For this review, take the finished solid that the model builds, in its own axes (mm). Face numbers are marked on the shaded views. A direction names the side the tool comes from. Coordinates: 2 decimals unless noted, no trailing zeros. Order: outer loops, then holes, each group sorted by start corner. A loop starts at its lowest first (then second) coordinate and runs counter-clockwise, first axis right, second up. Notation, with made-up numbers: (87, 7) - (139, 7) arc R21 ccw to (139, 33) - close; hole circle Ø11 at (-17, 34.25). An arc over 180 degrees is marked (long way). One line per item, written item: value. Start each with the question number.
(1) To check wall thickness, follow line 1 along X through (y, z) = (-1.4, 0.55); line 2 along X through (y, z) = (0.1, -0.4); line 3 along Y through (x, z) = (4.5, 0.4). State the ranges of each line that lie inside material, in increasing order.
(2) Consider section A-A on x = 3. Write out the cut boundary in (y, z), then the cut area to 3 significant figures.
(3) Clearance check with flat-ended pins moving along their axes: pin 1 (1.5 mm diameter, centred on x = 2, z = 0.5, fed in from -Y); pin 2 (0.6 mm diameter, centred on x = 0.5, z = -0.5, fed in from -Y); pin 3 (1.5 mm diameter, centred on x = 4, y = 1.5, fed in from -Z); pin 4 (1.3 mm diameter, centred on x = 0.5, y = -0.5, fed in from -Z). State where each tip first meets the part, or that it passes through.
(4) For the marked faces 1, 2 and 3, list the 3-axis set-ups (+Z, -Z, +X, -X, +Y, -Y) from which the entire face can be reached by the end or side of a thin tool; tool diameter is ignored.
(5) Consider section B-B on x = 5.75. Write out the cut boundary in (y, z), then the cut area to 3 significant figures.
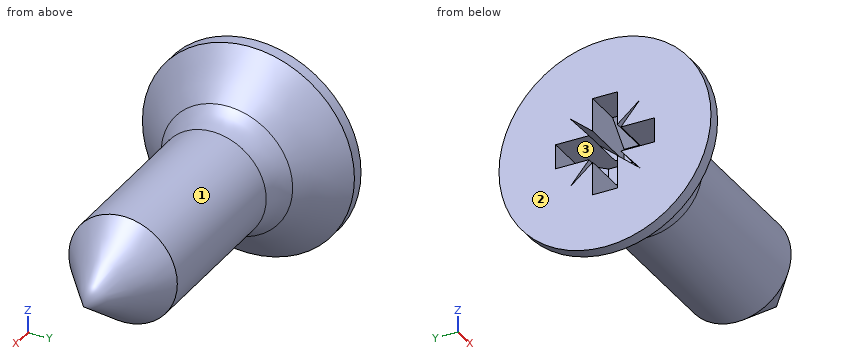
Solid Edge part; units mm, degrees
sketch "Sketch1" plane through (0, 0, 0) normal (0, 0, 1) x (1, 0, 0)
  line L0 (0, 0) -> (0, 2.15)
  line L1 (0, 2.15) -> (0.25, 2.15)
  line L2 (0.25, 2.15) -> (1.0657, 1.3343)
  arc A0 (1.0657, 1.3343) -> (1.6314, 1.1) centre (1.6314, 1.9) ccw
  line L3 (1.6314, 1.1) -> (5, 1.1)
  line L4 (5, 1.1) -> (6.5, 0)
  line L5 (6.5, 0) -> (0, 0)
revolve "RevolvedProtrusion1" add sketch "Sketch1" angle 360 about axis through (10.8, 0, 0) along (-1, 0, 0)
cosmetic_thread "Thread_1" thread depth 2.9
sketch "Sketch2" plane through (0, 0, 0) normal (0, 0, 1) x (1, 0, 0)
  line L0 (0, -1) -> (0.7667, -1)
  line L1 (0.7667, -1) -> (1.2, -0.5667)
  line L2 (1.2, -0.5667) -> (1.2, 0.5667)
  line L3 (1.2, 0.5667) -> (0.7667, 1)
  line L4 (0.7667, 1) -> (0, 1)
  line L5 (0, 1) -> (0, -1)
extrude "ExtrudedCutout_1" cut sketch "Sketch2" against normal blind 0.25 and the other way blind 0.25
sketch "Sketch3" plane through (0, 0, 0) normal (0, -1, 0) x (1, 0, 0)
  line L0 (-0.1, 1) -> (0.7567, 1)
  line L1 (0.7567, 1) -> (1.19, 0.5667)
  line L2 (1.19, 0.5667) -> (1.19, -0.5667)
  line L3 (1.19, -0.5667) -> (0.7567, -1)
  line L4 (0.7567, -1) -> (-0.1, -1)
  line L5 (-0.1, -1) -> (-0.1, 1)
extrude "ExtrudedCutout_2" cut sketch "Sketch3" against normal blind 0.25 and the other way blind 0.25
sketch "Sketch4" plane through (0, 0, 0) normal (-1, 0, 0) x (0, -1, 0)
  line L0 (0.7071, 0.7071) -> (0, 0.1138)
  line L1 (0, 0.1138) -> (-0.7071, 0.7071)
  line L2 (-0.7071, 0.7071) -> (-0.1138, 0)
  line L3 (-0.1138, 0) -> (-0.7071, -0.7071)
  line L4 (-0.7071, -0.7071) -> (0, -0.1138)
  line L5 (0, -0.1138) -> (0.7071, -0.7071)
  line L6 (0.7071, -0.7071) -> (0.1138, 0)
  line L7 (0.1138, 0) -> (0.7071, 0.7071)
extrude "ExtrudedCutout_3" cut sketch "Sketch4" against normal blind 1
properties part number "bene_inox_212408-2,2X6,5"
Geometry check:
1. line 1: x = 0 to 0.9
1. line 2: x = 1.19 to 5.94
1. line 3: y = -1.02 to 1.02
2. outline: circle Ø2.2 at (0, 0)
2. area: 3.80 mm^2
3. pin 1: stops at y = -1.15
3. pin 2: stops at y = -2.12
3. pin 3: stops at z = -0.8
3. pin 4: stops at z = -2.15
4. face 1: +X
4. face 2: +Z, -Z, -X, +Y, -Y
4. face 3: -X
5. outline: circle Ø1.1 at (0, 0)
5. area: 0.950 mm^2
